```python
from build123d import *

# Parameters (mm, degrees)
SKETCH1_W                                            = 60
SKETCH1_H                                            = 125
BOSS_EXTRUDE1_DEPTH                                  = 10
SKETCH2_R                                            = 9.5
BOSS_EXTRUDE2_DEPTH                                  = 25
CSK_FOR_M5_COUNTERSUNK_RAISED_HEAD_SCREW_D           = 5.5
CSK_FOR_M5_COUNTERSUNK_RAISED_HEAD_SCREW_CSINK_D     = 10.4
CSK_FOR_M5_COUNTERSUNK_RAISED_HEAD_SCREW_CSINK_ANGLE = 90


with BuildPart() as part:
    # Sketch1 → Boss-Extrude1 (new body)
    with BuildSketch(Plane(origin=(0, 0, 0), x_dir=(1, 0, 0), z_dir=(0, 1, 0))):
        with Locations((30, 62.5)):
            Rectangle(SKETCH1_W, SKETCH1_H)
    extrude(amount=BOSS_EXTRUDE1_DEPTH)

    # Sketch2 → Boss-Extrude2 (add)
    with BuildSketch(Plane(origin=(0, 0, -125), x_dir=(-1, 0, 0), z_dir=(0, 0, -1))):
        with BuildLine():
            Line((-60, 10), (0, 10))
            Line((0, 10), (0, 64))
            ThreePointArc((0, 64), (-30, 94), (-60, 64))
            Line((-60, 64), (-60, 10))
        make_face()
        with Locations((-30, 64)):
            Circle(SKETCH2_R, mode=Mode.SUBTRACT)
    extrude(amount=-BOSS_EXTRUDE2_DEPTH)

    # CSK for M5 Countersunk Raised Head Screw1 (through all)
    with Locations(Plane(origin=(30, 10, -50), x_dir=(0, 0, 1), z_dir=(0, 1, 0))):
        with Locations((0, 0)):
            CounterSinkHole(CSK_FOR_M5_COUNTERSUNK_RAISED_HEAD_SCREW_D / 2, CSK_FOR_M5_COUNTERSUNK_RAISED_HEAD_SCREW_CSINK_D / 2, counter_sink_angle=CSK_FOR_M5_COUNTERSUNK_RAISED_HEAD_SCREW_CSINK_ANGLE)


solid = part.part
```
Here's how the part is built. I have some questions about the finished solid (model axes, mm). A direction names the side the tool comes from. Coordinates: 2 decimals unless noted, no trailing zeros. Order: outer loops, then holes, each group sorted by start corner. A loop starts at its lowest first (then second) coordinate and runs counter-clockwise, first axis right, second up. Notation, with made-up numbers: M 52.5,-16 L 57.5,-16 A20 ccw 57.5,-7 Z; hole C 17,65 d4. An arc over 180 degrees is marked long. Answer as a JSON object with one key per item and string values. Group by question number.
(1) I need wall thicknesses on probe 1 along Y at (x, z) = (30, -112.5); probe 2 along Z at (x, y) = (30, 5); probe 3 along Z at (x, y) = (16, 75.5). Which ranges of each line are inside material? Lowest first, please.
(2) Suppose I cut it at D-D, the plane z = -10.5. Please give me the cut outline in (x, y).
(3) Suppose I cut it at B-B, the plane x = 30. Please give me the cut outline in (y, z), then the cut area to 3 significant figures.
(4) If we mould it in two halves opening along X, with no side actions, what happens to faces 1 (the face through (30, 53, -100)), 2 (the face through (31.24, 73.42, -112.68)), 3 (the face through (60, 8, -91))? For each: released by +X, released by -X, zero draft, split by the parting line, or undercut.
(5) Suppose I cut it at C-C, the plane x = 49. Please give me the cut outline in (y, z).
(6) Which directions (+Z, -Z, +X, -X, +Y, -Y) give clear straight access to the entire face, cutting with the end or side of a thin tool? Please do faces 4 (the face through (23, 10, -51)), 5 (the face through (30, 0, -63)).
(7) For pin 1 (3 mm diameter, centred on x = 17.5, z = -96.5, fed in from +Y); pin 2 (8 mm diameter, centred on y = 26, z = -95, fed in from -X) (3 decimals); pin 3 (1 mm diameter, centred on x = 42, z = -16, fed in from -Y); pin 4 (24.5 mm diameter, centred on x = 30, y = 64, fed in from +Z), each with a flat end and sliding along its axis, tell me the tip position at first contact or that it passes through.
(8) Suppose I cut it at A-A, the plane z = -50. Please give me the cut outline in (x, y).
Values found:
{
 "1": {"probe 1": "y = 0 to 54.5, 73.5 to 94", "probe 2": "z = -125 to -52.75, -47.25 to 0", "probe 3": "z = -125 to -100"},
 "2": {"outline": "M 0,0 L 60,0 L 60,10 L 0,10 Z"},
 "3": {"outline": "M 0,-125 L 54.5,-125 L 54.5,-100 L 10,-100 L 10,-55.2 L 7.55,-52.75 L 0,-52.75 Z; M 0,-47.25 L 7.55,-47.25 L 10,-44.8 L 10,0 L 0,0 Z; M 73.5,-125 L 94,-125 L 94,-100 L 73.5,-100 Z", "area": "2,810 mm^2"},
 "4": {"face 1": "zero draft", "face 2": "undercut", "face 3": "released by +X"},
 "5": {"outline": "M 0,-125 L 87.22,-125 L 87.22,-100 L 10,-100 L 10,0 L 0,0 Z"},
 "6": {"face 4": "+Z, +X, -X, +Y", "face 5": "+Z, -Z, +X, -X, -Y"},
 "7": {"pin 1": "stops at y = 10", "pin 2": "passes through", "pin 3": "stops at y = 0", "pin 4": "stops at z = -100"},
 "8": {"outline": "M 0,0 L 27.25,0 L 27.25,7.55 L 24.8,10 L 0,10 Z; M 32.75,0 L 60,0 L 60,10 L 35.2,10 L 32.75,7.55 Z"}
}
